The listing builds one solid part. Answer for the finished solid, in the listing's coordinates (mm). A direction names the side the tool comes from. Give positions to 0.01 mm unless a question says otherwise; leave off trailing zeros. Write each loop counter-clockwise with the first axis right and the second up, starting at its lowest first coordinate (ties: lowest second). Pieces come first, ordered by that corner, then holes. Notation, with made-up numbers: M 20.5,0.25 L 56.5,0.25 A18 ccw 56.5,13.25 Z; hole C 49,-9.75 d3. An arc over 180 degrees is marked long. Return JSON: item names as keys, results as strings.
from build123d import *

# Parameters (mm, degrees)
SKETCH_1_R      = 4.5
SKETCH_1_R_2    = 2
SKETCH_1_R_3    = 1.5
EXTRUDE_1_DEPTH = 1.5


with BuildPart() as part:
    # 草图1 → 凸台-拉伸1 (new body)
    with BuildSketch(Plane(origin=(0, 0, 0), x_dir=(1, 0, 0), z_dir=(0, 1, 0))):
        Polygon((20.023596815, 17.047193631), (20.023596815, 34), (15.976403185, 38.047193631), (15.976403185, 51), (12.476403185, 54.5), (12.476403185, 57), (12.476403185, 63.031398934), (9.023596815, 66.484205303), (9.023596815, 71.578592565), (12.476403185, 75.031398934), (12.476403185, 94.595844768), (8.976403185, 98.095844768), (8.976403185, 103.001457506), (12.476403185, 106.501457506), (12.476403185, 116.5), (8.976403185, 120), (-8.976403185, 120), (-12.476403185, 116.5), (-12.476403185, 106.501457506), (-8.976403185, 103.001457506), (-8.976403185, 98.095844768), (-12.476403185, 94.595844768), (-12.476403185, 75.031398934), (-9.023596815, 71.578592565), (-9.023596815, 66.484205303), (-12.476403185, 63.031398934), (-12.476403185, 57), (-12.476403185, 54.5), (-15.976403185, 51), (-15.976403185, 38.047193631), (-20.023596815, 34), (-20.023596815, 17.047193631), (-15.976403185, 13), (-15.976403185, 3.452806369), (-12.476403185, -0.047193631), (-12.476403185, -9.952806369), (-15.976403185, -13.452806369), (-15.976403185, -43.547193631), (-12.523596815, -47), (12.523596815, -47), (15.976403185, -43.547193631), (15.976403185, -13.452806369), (12.476403185, -9.952806369), (12.476403185, -0.047193631), (15.976403185, 3.452806369), (15.976403185, 13), align=None)
        with Locations(Location((0, 25.5, 0), (0, 0, 270))):
            Circle(SKETCH_1_R, mode=Mode.SUBTRACT)
        with Locations(Location((8, 25.5, 0), (0, 0, 270))):
            Circle(SKETCH_1_R_2, mode=Mode.SUBTRACT)
        with Locations(Location((0, 16, 0), (0, 0, 270))):
            Circle(SKETCH_1_R_2, mode=Mode.SUBTRACT)
        with Locations(Location((-8, 25.5, 0), (0, 0, 270))):
            Circle(SKETCH_1_R_2, mode=Mode.SUBTRACT)
        with Locations(Location((0, 35, 0), (0, 0, 270))):
            Circle(SKETCH_1_R_2, mode=Mode.SUBTRACT)
        with Locations(Location((11, 3.5, 0), (0, 0, 270))):
            Circle(SKETCH_1_R_3, mode=Mode.SUBTRACT)
        with Locations(Location((11, 47.5, 0), (0, 0, 270))):
            Circle(SKETCH_1_R_3, mode=Mode.SUBTRACT)
        with Locations(Location((-11, 47.5, 0), (0, 0, 90))):
            Circle(SKETCH_1_R_3, mode=Mode.SUBTRACT)
        with Locations(Location((-11, 3.5, 0), (0, 0, 90))):
            Circle(SKETCH_1_R_3, mode=Mode.SUBTRACT)
        with Locations(Location((11, -13.5, 0), (0, 0, 270))):
            Circle(SKETCH_1_R_3, mode=Mode.SUBTRACT)
        with Locations(Location((11, -43.5, 0), (0, 0, 270))):
            Circle(SKETCH_1_R_3, mode=Mode.SUBTRACT)
        with Locations(Location((-11, -13.5, 0), (0, 0, 90))):
            Circle(SKETCH_1_R_3, mode=Mode.SUBTRACT)
        with Locations(Location((-11, -43.5, 0), (0, 0, 90))):
            Circle(SKETCH_1_R_3, mode=Mode.SUBTRACT)
    extrude(amount=EXTRUDE_1_DEPTH)


solid = part.part
Item 1: Find the intervals of material crossed by line 1 (X direction, y = 0.8, z = -3.5); line 2 (Z direction, x = -3.5, y = 0.65); line 3 (X direction, y = 0.25, z = -113), in increasing order.
Geometry results:
{"line 1": "x = -15.98 to -12.5, -9.5 to 9.5, 12.5 to 15.98", "line 2": "z = -120 to -28.33, -22.67 to 47", "line 3": "x = -12.48 to 12.48"}
Item 2: A cutting plane is placed at D-D, the plane x = 14. Write down the section's boundary in (y, z).
Geometry results:
{"outline": "M 0,-52.98 L 1.5,-52.98 L 1.5,-1.48 L 0,-1.48 Z; M 0,11.48 L 1.5,11.48 L 1.5,45.52 L 0,45.52 Z"}
Item 3: A cutting plane is placed at C-C, the plane z = -47.5. Write down the section's boundary in (x, y).
Geometry results:
{"outline": "M -15.98,0 L -12.5,0 L -12.5,1.5 L -15.98,1.5 Z; M -9.5,0 L 9.5,0 L 9.5,1.5 L -9.5,1.5 Z; M 12.5,0 L 15.98,0 L 15.98,1.5 L 12.5,1.5 Z"}
Item 4: A cutting plane is placed at A-A, the plane x = 0. Write down the section's boundary in (y, z).
Geometry results:
{"outline": "M 0,-120 L 1.5,-120 L 1.5,-37 L 0,-37 Z; M 0,-33 L 1.5,-33 L 1.5,-30 L 0,-30 Z; M 0,-21 L 1.5,-21 L 1.5,-18 L 0,-18 Z; M 0,-14 L 1.5,-14 L 1.5,47 L 0,47 Z"}
Item 5: Which of the six approach directions +Z, -Z, +X, -X, +Y, -Y give full straight-line access (tool end or side, diameter ignored) to faces 1 (the flat face through (-10.73, 0.74, -64.78)), 2 (the flat face through (10.726, 0.74, -73.281)), 3 (the flat face through (17.972, 0.74, -14.995))?
Geometry results:
{"face 1": "-X, +Y, -Y", "face 2": "+X, +Y, -Y", "face 3": "+Z, +X, +Y, -Y"}
Item 6: Determine the mould class of faces 4 (the cylindrical face through (11, 1, 42)), 5 (the flat face through (14.251, 0.74, -52.726)), 6 (the flat face through (0, 0, -38)) for opening direction Z: +Z half, -Z half, draft (parallel to the pull), parting line (faces both ways), or undercut.
Geometry results:
{"face 4": "undercut", "face 5": "-Z half", "face 6": "draft"}
Item 7: A cutting plane is placed at B-B, the plane z = -25.5. Write down the section's boundary in (x, y), plus the area to 3 significant figures.
Geometry results:
{"outline": "M -20.02,0 L -10,0 L -10,1.5 L -20.02,1.5 Z; M -6,0 L -4.5,0 L -4.5,1.5 L -6,1.5 Z; M 4.5,0 L 6,0 L 6,1.5 L 4.5,1.5 Z; M 10,0 L 20.02,0 L 20.02,1.5 L 10,1.5 Z", "area": "34.6 mm2"}
Item 8: Given pin 1 Ø2.5 at (x, z) = (0, -35) entering from -Y, flat-ended and moving along its own axis, determine where the tip first touches the part or whether it passes through.
Geometry results:
{"pin 1": "passes through"}
